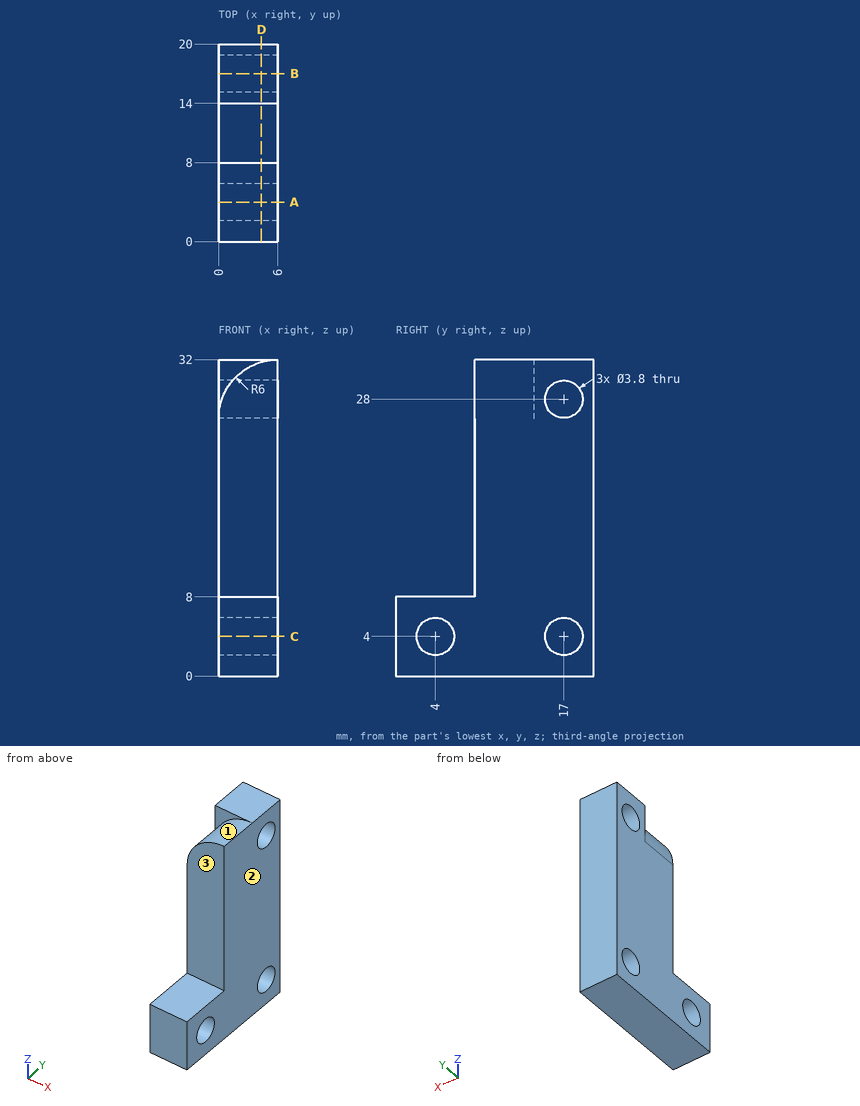
Check sheet for the drawn part. Datum: minimum x, y, z corner. Units: mm. A direction names the side the tool comes from. Coordinates: 2 decimals unless noted, no trailing zeros. Order: outer loops, then holes, each group sorted by start corner. A loop starts at its lowest first (then second) coordinate and runs counter-clockwise, first axis right, second up. Notation, with made-up numbers: M 18,53.25 L 51,53.25 A20 ccw 51,60.25 Z; hole C 8,38 d9. An arc over 180 degrees is marked long. One line per item, written item: value. Start each with the question number.
Item 1: Sectioned sample at B-B (y = 17). Enter the section's corners in (x, z), then the cut area to 3 significant figures.
Item 2: Access from +Z, -Z, +X, -X, +Y, -Y to the whole of each face (thin tool, end or side, straight path). Record for the marked faces 1, 2 and 3.
Item 3: Sectioned sample at D-D (x = 4.35). Enter the section's corners in (y, z).
Item 4: Gauge pin test, flat ends, axial feed: pin 1 (3 mm diameter, centred on x = 4.5, y = 3, fed in from +Z); pin 2 (2.5 mm diameter, centred on y = 17, z = 4, fed in from +X); pin 3 (3 mm diameter, centred on x = 2.5, z = 22, fed in from -Y). Record the tip position at first contact, or that the pin passes through.
Item 5: Sectioned sample at A-A (y = 4). Enter the section's corners in (x, z).
Item 6: Sectioned sample at C-C (z = 4). Enter the section's corners in (x, y), then the cut area to 3 significant figures.
Item 7: Scan lines: probe 1 along Z at (x, y) = (2.5, 17); probe 2 along Y at (x, z) = (3.65, 4); probe 3 along Y at (x, z) = (4.55, 28). Record each from-to range of solid material in increasing order.
Conclusion:
1. outline: M 0,0 L 6,0 L 6,2.1 L 0,2.1 Z; M 0,5.9 L 6,5.9 L 6,26.1 L 0,26.1 Z; M 0,29.9 L 6,29.9 L 6,32 L 0,32 Z
1. area: 146 mm^2
2. face 1: +Z, -X, -Y
2. face 2: +Z, -Z, +X, +Y, -Y
2. face 3: +Z, +X, -X, -Y
3. outline: M 0,0 L 20,0 L 20,32 L 14,32 L 14,31.77 L 8,31.77 L 8,8 L 0,8 Z; hole C 4,4 d3.8; hole C 17,4 d3.8; hole C 17,28 d3.8
4. pin 1: stops at z = 8
4. pin 2: passes through
4. pin 3: stops at y = 8
5. outline: M 0,0 L 6,0 L 6,2.1 L 0,2.1 Z; M 0,5.9 L 6,5.9 L 6,8 L 0,8 Z
6. outline: M 0,0 L 6,0 L 6,2.1 L 0,2.1 Z; M 0,5.9 L 6,5.9 L 6,15.1 L 0,15.1 Z; M 0,18.9 L 6,18.9 L 6,20 L 0,20 Z
6. area: 74.4 mm^2
7. probe 1: z = 0 to 2.1, 5.9 to 26.1, 29.9 to 32
7. probe 2: y = 0 to 2.1, 5.9 to 15.1, 18.9 to 20
7. probe 3: y = 8 to 15.1, 18.9 to 20
